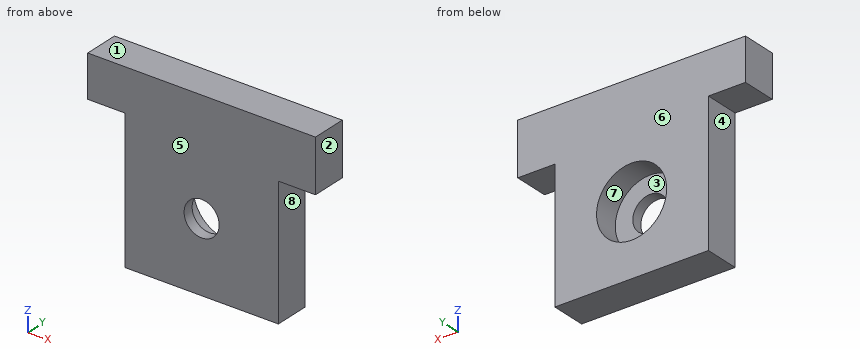
from build123d import *

# Parameters (mm, degrees)
BOSS_EXTRUDE1_DEPTH = 10
SKETCH2_R           = 10
CUT_EXTRUDE2_DEPTH  = 7
SKETCH5_R           = 5
CUT_EXTRUDE3_DEPTH  = 4


with BuildPart() as part:
    # Sketch1 → Boss-Extrude1 (new body)
    with BuildSketch(Plane(origin=(0, 0, 0), x_dir=(1, 0, 0), z_dir=(0, 1, 0))):
        Polygon((-21.887133372, 52), (21.887133372, 51.952432224), (21.887133372, 14.952432224), (32.458561943, 14.952432224), (32.458561943, 0), (-32.458561943, 0), (-32.458561943, 12), (-21.887133372, 12), align=None)
    extrude(amount=BOSS_EXTRUDE1_DEPTH)

    # Sketch2 → Cut-Extrude2 (cut)
    with BuildSketch(Plane(origin=(0, 10, 0), x_dir=(1, 0, 0), z_dir=(0, 1, 0))):
        with Locations((0, 32)):
            Circle(SKETCH2_R)
    extrude(amount=-CUT_EXTRUDE2_DEPTH, mode=Mode.SUBTRACT)

    # Sketch5 → Cut-Extrude3 (cut, through all)
    with BuildSketch(Plane(origin=(0, 3, 0), x_dir=(1, 0, 0), z_dir=(0, 1, 0))):
        with Locations((0, 32)):
            Circle(SKETCH5_R)
    extrude(amount=-CUT_EXTRUDE3_DEPTH, mode=Mode.SUBTRACT)


solid = part.part
Model file for the job. Use its own axes, mm. Face numbers are marked on the shaded views. A direction names the side the tool comes from. Coordinates: 2 decimals unless noted, no trailing zeros. Order: outer loops, then holes, each group sorted by start corner. A loop starts at its lowest first (then second) coordinate and runs counter-clockwise, first axis right, second up. Notation, with made-up numbers: (-24, 18.25) -> (24, 18.25) arc R22 cw to (24, 51.25) -> close; hole circle Ø10 at (57, 34.25). An arc over 180 degrees is marked (long way). Return JSON: item names as keys, results as strings. Group by question number.
Item 1: Saw through at C-C on x = 2.5. Write the cut outline in (y, z), then the cut area to 3 significant figures.
Item 2: Saw through at A-A on z = -32. Write the cut outline in (x, y), then the cut area to 3 significant figures.
Item 3: Saw through at B-B on y = 7.75. Write the cut outline in (x, z).
Item 4: Pull direction Z, two halves, no side cores. Call the marked faces 1, 2 and 3: pulls with the +Z half, pulls with the -Z half, needs draft (parallel to the pull), parting line crosses it, or undercut.
Item 5: Saw through at D-D on z = -23.5. Write the cut outline in (x, y), then the cut area to 3 significant figures.
Item 6: Flat gauge pins, fed straight in: P1, Ø6, axis at y = 2.5, z = -23, coming from the +X side; P2, Ø2, axis at y = 1.5, z = -35, coming from the -X side; P3, Ø9, axis at x = 0, z = -32, coming from the -Y side (1 decimal); P4, Ø4, axis at x = 0, y = 5, coming from the -Z side. Where does each tip first touch, or does it go through?
Item 7: Tool access for the marked faces 4, 5, 6, 7 and 8: list every direction of +Z, -Z, +X, -X, +Y, -Y with a clear straight run to the whole face (end or side of a thin tool).
Item 8: Wall check: line 1 along X through (y, z) = (8, -32); line 2 along X through (y, z) = (1.35, -32); line 3 along Z through (x, y) = (-28, 3.5). Give the ranges that are in metal, low to high. Write a range as [from, to].
Values found:
{
 "1": {"outline": "(0, -51.97) -> (10, -51.97) -> (10, -41.68) -> (3, -41.68) -> (3, -36.33) -> (0, -36.33) -> close; (0, -27.67) -> (3, -27.67) -> (3, -22.32) -> (10, -22.32) -> (10, 0) -> (0, 0) -> close", "area": "358 mm2"},
 "2": {"outline": "(-21.89, 0) -> (-5, 0) -> (-5, 3) -> (-10, 3) -> (-10, 10) -> (-21.89, 10) -> close; (5, 0) -> (21.89, 0) -> (21.89, 10) -> (10, 10) -> (10, 3) -> (5, 3) -> close", "area": "268 mm2"},
 "3": {"outline": "(-32.46, -12) -> (-21.89, -12) -> (-21.89, -52) -> (21.89, -51.95) -> (21.89, -14.95) -> (32.46, -14.95) -> (32.46, 0) -> (-32.46, 0) -> close; hole circle Ø20 at (0, -32)"},
 "4": {"face 1": "pulls with the +Z half", "face 2": "needs draft", "face 3": "undercut"},
 "5": {"outline": "(-21.89, 0) -> (21.89, 0) -> (21.89, 10) -> (5.27, 10) -> (5.27, 3) -> (-5.27, 3) -> (-5.27, 10) -> (-21.89, 10) -> close", "area": "364 mm2"},
 "6": {"P1": "stops at x = 21.89", "P2": "stops at x = -21.89", "P3": "passes through", "P4": "stops at z = -51.98"},
 "7": {"face 4": "-Z, -X, +Y, -Y", "face 5": "+Z, -Z, +X, -X, -Y", "face 6": "+Z, -Z, +X, -X, +Y", "face 7": "+Y", "face 8": "-Z, +X, +Y, -Y"},
 "8": {"line 1": "x = [-21.89, -10], [10, 21.89]", "line 2": "x = [-21.89, -5], [5, 21.89]", "line 3": "z = [-12, 0]"}
}
